```python
from build123d import *

# Parameters (mm, degrees)
F1_DEPTH = 47
F2_SIZE  = 1


with BuildPart() as f1:
    # F0 (on Top) → F1 (new body)
    with BuildSketch(Plane.XY):
        Polygon((0, -5.588235), (0, 0), (-95, 0), (-95, -5.588235), (-8, -5.588235), (-8, -3.352941), (-5, -3.352941), (-5, -5.588235), align=None)
        Polygon((-95, -5.588235), (-95, 0), (-190, 0), (-190, -5.588235), (-185, -5.588235), (-185, -3.352941), (-182, -3.352941), (-182, -5.588235), align=None)
    extrude(amount=F1_DEPTH)

    # F2
    f2_edges = [f1.edges().sort_by_distance(p)[0] for p in [
        (0, 0, 23.5),
        (-95, 0, 47),
        (-190, 0, 23.5),
        (-95, 0, 0),
    ]]
    chamfer(f2_edges, length=F2_SIZE)


solid = f1.part
```
For this review, take the finished solid that the model builds, in its own axes (mm). A direction names the side the tool comes from. Round coordinates to 2 decimals unless told otherwise and drop trailing zeros. Write each loop counter-clockwise with the first axis right and the second up, starting at its lowest first coordinate (ties: lowest second). Pieces come first, ordered by that corner, then holes. Notation, with made-up numbers: (35, -11.75) - (57, -11.75) arc R16 cw to (57, 2.25) - close; hole circle Ø7 at (-7.5, 82.25). An arc over 180 degrees is marked (long way). Answer as CSV lines item,"result". Start each with the question number.
(1) Add section A-A, the plane y = -4.45. State the section outline as (x, z) points.
(2) For line 1 (X direction, y = -3.8, z = 13); line 2 (Z direction, x = -50, y = -0.25); line 3 (X direction, y = -0.25, z = 24.5), list the stretches that pass through material, from the lowest coordinate up.
(3) Mouldability with a two-part tool opening along X and no side actions: class faces 1 (the flat face through (0, -3, 23)), 2 (the flat face through (-96, -3, 0)), 3 (the flat face through (-7, -3.353, 23)) as +X half, -X half, draft (parallel to the pull), parting line (faces both ways), or undercut.
(4) For pin 1 (2 mm diameter, centred on x = -21.5, y = -1.5, fed in from -Z); pin 2 (0.9 mm diameter, centred on x = -183.5, z = 13.5, fed in from -Y), all flat-tipped, find the tip position at first contact; note any pin that passes through.
(5) Machinability: for faces 4 (the flat face through (-184, -3.353, 23)), 5 (the flat face through (-96, -5.588, 23)), which of the approach directions +Z, -Z, +X, -X, +Y, -Y give a long, thin tool a straight path to every point of the face, cutting with its end or side? Answer none if there is none.
From the geometry:
1,outline,"(-190, 0) - (-185, 0) - (-185, 47) - (-190, 47) - close; (-182, 0) - (-8, 0) - (-8, 47) - (-182, 47) - close; (-5, 0) - (0, 0) - (0, 47) - (-5, 47) - close"
2,line 1,"x = -190 to -185, -182 to -8, -5 to 0"
2,line 2,"z = 0.75 to 46.25"
2,line 3,"x = -189.25 to -0.75"
3,face 1,"+X half"
3,face 2,"draft"
3,face 3,"undercut"
4,pin 1,"stops at z = 0"
4,pin 2,"stops at y = -3.35"
5,face 4,"+Z, -Z, -Y"
5,face 5,"+Z, -Z, +X, -X, -Y"
